Autodesk Inventor part; units mm, degrees
ref_plane "Work Plane1" through (25, 0, 0) normal (1, 0, 0) x (0, 1, 0)
ref_plane "Work Plane2" through (0, 0, 60) normal (0, 0, 1) x (1, 0, 0)
ref_plane "XZ Plane" through (0, 0, 0) normal (0, 1, 0) x (-1, 0, 0)
ref_plane "Work Plane1" through (25, 0, 0) normal (1, 0, 0) x (0, 1, 0)
ref_plane "Work Plane2" through (0, 0, 60) normal (0, 0, 1) x (1, 0, 0)
sketch "Sketch1" plane through (0, 0, 0) normal (0, 1, 0) x (-1, 0, 0)
  line L0 (0, 0) -> (-50, 0)
  line L1 (-50, 0) -> (-50, 120)
  line L2 (-50, 120) -> (0, 120)
  line L3 (0, 120) -> (0, 0)
  line L4 (-18.5, 108.5) -> (-31.5, 108.5)
  line L5 (-31.5, 108.5) -> (-31.5, 11.5)
  line L6 (-31.5, 11.5) -> (-18.5, 11.5)
  line L7 (-18.5, 11.5) -> (-18.5, 108.5)
  dimension "d0" = 50
  dimension "d1" = 120
  dimension "d2" = 13
  dimension "d3" = 97
  dimension "d4" = 11.5
  dimension "d5" = 18.5
extrude "Extrusion1" add sketch "Sketch1" along normal blind 3
sketch "Sketch2" plane through (0, 0, 0) normal (0, -1, 0) x (1, 0, 0)
  line L0 (42.5, 115) -> (7.5, 115)
  line L1 (7.5, 115) -> (7.5, 5)
  line L2 (7.5, 5) -> (42.5, 5)
  line L3 (42.5, 5) -> (42.5, 115)
  line L4 (50, 0) -> (0, 0)
  line L5 (50, 120) -> (50, 0)
  line L6 (0, 0) -> (0, 120)
  line L7 (0, 120) -> (50, 120)
  dimension "d8" = 35
  dimension "d9" = 110
  dimension "d14" = 7.5
  dimension "d15" = 5
extrude "Extrusion2" add sketch "Sketch2" along normal blind 15 contours L3 L2 L1 L0
sketch "Sketch4" plane through (0, 3, 0) normal (0, 1, 0) x (1, 0, 0)
  line L0 (0, -120) -> (50, -120)
  line L1 (0, -120) -> (50, -120)
  line L2 (50, -120) -> (50, 0)
  line L3 (50, 0) -> (0, 0)
  line L4 (0, 0) -> (0, -120)
  line L5 (18.5, -11.5) -> (31.5, -11.5)
  line L6 (18.5, -108.5) -> (31.5, -108.5)
  line L7 (31.5, -11.5) -> (18.5, -11.5)
  line L8 (18.5, -108.5) -> (18.5, -11.5)
  line L9 (18.5, -67.5) -> (22, -67.5)
  line L10 (22, -67.5) -> (22, -52.5)
  line L11 (22, -52.5) -> (18.5, -52.5)
  line L12 (18.5, -52.5) -> (18.5, -67.5)
  line L13 (31.5, -11.5) -> (31.5, -108.5)
  line L14 (31.5, -67.5) -> (28, -67.5)
  line L15 (28, -67.5) -> (28, -52.5)
  line L16 (28, -52.5) -> (31.5, -52.5)
  line L17 (31.5, -52.5) -> (31.5, -67.5)
  line L18 (18.5, -67.5) -> (18.5, -108.5)
  line L19 (31.5, -67.5) -> (31.5, -108.5)
  line L20 (31.5, -52.5) -> (31.5, -11.5)
  line L21 (18.5, -52.5) -> (18.5, -11.5)
  point P0 (0, 0)
  dimension "d16" = 15
  dimension "d17" = 3.5
  dimension "d18" = 3.5
  dimension "d19" = 41
extrude "Extrusion3" add sketch "Sketch4" along normal blind 2 contours L4 L3 L2 L0 | L11 L10 L9 L8 | L13 L14 L15 L16
sketch "Sketch6" plane through (18.5, 0, 108.5) normal (1, 0, 0) x (0, 0, -1)
  point P0 (108.5, 0)
  point P1 (3.711, 1.7158)
hole "Hole1" at (18.5, 1.7158, 104.789) direction (-1, 0, 0) diameter 2 end through all
pattern_linear "Rectangular Pattern1" count 12 spacing 8 along (0, 0, -1) of "Hole1"
mirror "Mirror1" about plane through (25, 0, 0) normal (1, 0, 0) of "Hole1", "Rectangular Pattern1"
sketch "Sketch8" plane through (31.5, 0, 108.5) normal (0, 0, -1) x (-1, 0, 0)
  point P0 (31.5, 0)
  point P1 (11.368, 2.2274)
hole "Hole2" at (20.132, 2.2274, 108.5) direction (0, 0, 1) diameter 2 end through all
pattern_linear "Rectangular Pattern2" count 3 spacing 5 along (1, 0, 0) of "Hole2"
mirror "Mirror2" about plane through (0, 0, 60) normal (0, 0, 1) of "Hole2", "Rectangular Pattern2"
properties part number "dhillg25_P2_Milestone3"
Geometry: final body of the model. Coordinates: model frame, mm. A direction names the side the tool comes from. Round coordinates to 2 decimals unless told otherwise and drop trailing zeros. Order: outer loops, then holes, each group sorted by start corner. A loop starts at its lowest first (then second) coordinate and runs counter-clockwise, first axis right, second up. Notation, with made-up numbers: M 67.5,79.5 L 104.5,79.5 A15 ccw 104.5,96.5 Z; hole C 46.5,18 d6. An arc over 180 degrees is marked long. Use one line per item in the form item = value. Start each with the question number.
Q1. Access query for faces 4 (the face through (40.88, 1.333, 103.865)), 5 (the face through (20, 4, 67.5)). Directions: +Z, -Z, +X, -X, +Y, -Y. A direction counts if a zero-diameter tool reaches every point of the face in a straight line with its end or side. Return the directions, or none.
Q2. Material intervals for line 1 (Z direction, x = 29, y = 4); line 2 (X direction, y = 3, z = 47.5); line 3 (Z direction, x = 31.5, y = -7.75), sorted ascending. Write a range as [from, to].
Q3. Cut plane A-A (z = 91). Return loops of the section in (x, y), and give its area (3 significant figures).
Q4. Pin query (flat end, axial travel): pin 1 Ø1 at (y, z) = (-7.5, 94) entering from +X. Return the tip coordinate at first contact, or that it passes through.
Q5. Cut plane B-B (x = 34). Count the separate pieces of the cut face and the enclosed holes in it, and give its area (3 significant figures).
Q6. Cut plane C-C (y = -8.75). Return loops of the section in (x, z), and give its area (3 significant figures).
Q7. Mould query, pull axis X, two halves, no side actions, for faces 1 (the face through (31.123, 2.097, 5.67)), 2 (the face through (40.88, 1.76, 41.79)), 3 (the face through (42.5, -7, 59)). Classes: +X half, -X half, draft (parallel to the pull), parting line (faces both ways), or undercut.
Geometry results:
q1.face_4 = +X, -X
q1.face_5 = +Y
q2.line_1 = [0, 11.5], [52.5, 67.5], [108.5, 120]
q2.line_2 = [0, 18.5], [31.5, 50]
q2.line_3 = [5, 115]
q3.outline = M 0,0 L 7.5,0 L 7.5,-15 L 42.5,-15 L 42.5,0 L 50,0 L 50,5 L 31.5,5 L 31.5,0 L 18.5,0 L 18.5,5 L 0,5 Z
q3.area = 710 mm^2
q4.pin_1 = 42.5
q5.separate_pieces = 1
q5.enclosed_holes = 12
q5.area = 2,210 mm^2
q6.outline = M 7.5,5 L 42.5,5 L 42.5,115 L 7.5,115 Z
q6.area = 3,850 mm^2
q7.face_1 = undercut
q7.face_2 = draft
q7.face_3 = +X half
